Autodesk Inventor part; units mm, degrees
ref_plane "YZ Plane" through (0, 0, 0) normal (1, 0, 0) x (0, 1, 0)
ref_plane "XZ Plane" through (0, 0, 0) normal (0, 1, 0) x (-1, 0, 0)
ref_plane "XY Plane" through (0, 0, 0) normal (0, 0, 1) x (1, 0, 0)
sketch "スケッチ1" plane through (0, 0, 0) normal (1, 0, 0) x (0, 1, 0)
  line L0 (5, 5) -> (-5, 5)
  line L1 (-5, 5) -> (-5, -5)
  line L2 (-5, -5) -> (5, -5)
  line L3 (5, -5) -> (5, 5)
  line L4 (4, 4) -> (-4, 4)
  line L5 (-4, 4) -> (-4, -4)
  line L6 (-4, -4) -> (4, -4)
  line L7 (4, -4) -> (4, 4)
  point P0 (0, 0)
  dimension "d0" = 1
  dimension "d1" = 1
  dimension "d2" = 1
  dimension "d3" = 1
  dimension "d4" = 10
  dimension "d5" = 10
  dimension "d6" = 5
  dimension "d7" = 5
extrude "押し出し1" add sketch "スケッチ1" along normal blind 40
sketch "スケッチ2" plane through (0, -5, 5) normal (0, 0, 1) x (1, 0, 0)
  circle A0 centre (5, 5) radius 1.5
  circle A1 centre (25, 5) radius 1.5
  line L0 (0, 10) -> (0, 0)
  line L1 (0, 0) -> (40, 0)
  line L2 (40, 10) -> (40, 0)
  point P0 (0, 5)
  dimension "d10" = 5
  dimension "d11" = 5
  dimension "d12" = 5
  dimension "d13" = 15
  dimension "d14" = 3
  dimension "d15" = 3
extrude "押し出し2" cut sketch "スケッチ2" against normal blind 30
sketch "スケッチ3" plane through (0, -5, -5) normal (0, -1, 0) x (1, 0, 0)
  circle A0 centre (35, 5) radius 1.5
  line L0 (40, 10) -> (40, 0)
  line L1 (0, 0) -> (40, 0)
  point P0 (0, 5)
  dimension "d18" = 5
  dimension "d19" = 5
  dimension "d20" = 3
extrude "押し出し3" cut sketch "スケッチ3" against normal blind 30
properties part number "モーターパーツ２" material "アルミニウム 6061"
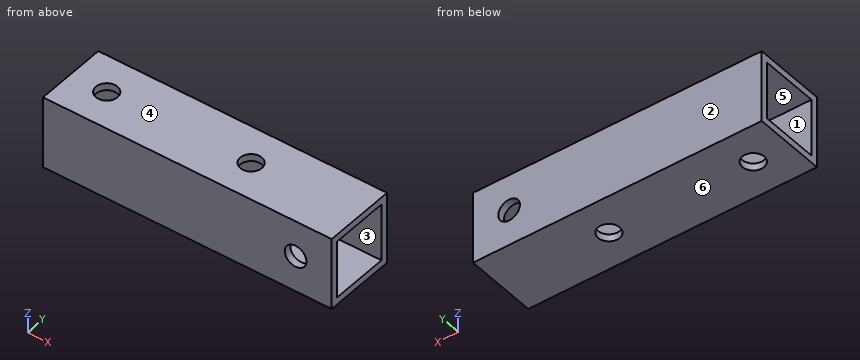
Can you work these out from the model? Positions are in its coordinate system, mm. Face numbers are marked on the shaded views. A direction names the side the tool comes from. Give positions to 0.01 mm unless a question says otherwise; leave off trailing zeros. Loops run counter-clockwise (first coordinate to the right, second up) from the corner with the lowest first, then second, coordinate; pieces in that order, holes last. Notation, with made-up numbers: M 14.25,59 L 64.25,59 A14 ccw 64.25,79 Z; hole C 39,7.5 d11. An arc over 180 degrees is marked long. Use CSV: the item, a comma, the result in double quotes. Start each with the question number.
1. If we mould it in two halves opening along Y, with no side actions, what happens to the marked faces 1, 2, 3 and 4? For each: released by +Y, released by -Y, zero draft, split by the parting line, or undercut.
2. Imagine slicing it at C-C, the plane x = 27. Write out the boundary of the cut face in (y, z).
3. Imagine slicing it at B-B, the plane z = -2.25. Write out the boundary of the cut face in (x, y), plus the area to 3 significant figures.
4. Imagine slicing it at A-A, the plane y = 0. Write out the boundary of the cut face in (x, z).
5. On a 3-axis mill with a long thin cutter (end or side, diameter ignored), from which of +Z, -Z, +X, -X, +Y, -Y can I reach the whole of each face in a straight line? I mean the marked faces 5 and 6. Say none if no direction works.
6. If I drill on L1, parallel to Z at x = 36.5, y = -3.5; L2, parallel to Y at x = 5, z = -4.65, over which ranges is the centre line in solid material (lowest first)?
Response values:
1,face 1,"undercut"
1,face 2,"released by +Y"
1,face 3,"undercut"
1,face 4,"zero draft"
2,outline,"M -5,-5 L 5,-5 L 5,5 L -5,5 Z; hole M -4,-4 L 4,-4 L 4,4 L -4,4 Z"
3,outline,"M 0,-5 L 40,-5 L 40,-4 L 0,-4 Z; M 0,4 L 40,4 L 40,5 L 0,5 Z"
3,area,"80.0 mm^2"
4,outline,"M 0,-5 L 3.5,-5 L 3.5,-4 L 0,-4 Z; M 0,4 L 3.5,4 L 3.5,5 L 0,5 Z; M 6.5,-5 L 23.5,-5 L 23.5,-4 L 6.5,-4 Z; M 6.5,4 L 23.5,4 L 23.5,5 L 6.5,5 Z; M 26.5,-5 L 40,-5 L 40,-4 L 26.5,-4 Z; M 26.5,4 L 40,4 L 40,5 L 26.5,5 Z"
5,face 5,"+X, -X"
5,face 6,"-Z, +X, -X, +Y, -Y"
6,L1,"-5 to -4, 4 to 5"
6,L2,"-5 to -1.5, 1.5 to 5"
